```python
from build123d import *

# Parameters (mm, degrees)
EXTRUDE_1_DEPTH             = 30
FILLET_3_R                  = 3
SKETCH_9_R                  = 5
CUT_EXTRUDE_5_DEPTH         = 64.837130412
CUT_EXTRUDE_6_DEPTH         = 27
PATTERN_CIRCULAR_1_COUNT    = 3
SKETCH_11_W                 = 20
SKETCH_11_H                 = 0.244863729
CUT_EXTRUDE_7_DEPTH         = 64.837130412
CUT_EXTRUDE_8_REACH         = 74.953
SKETCH_12_R                 = 1.5
HOLE_WIZARD_M3_1_AT_2_COUNT = 2
HOLE_WIZARD_M3_1_AT_2_PITCH = 24
PATTERN_CIRCULAR_2_COUNT    = 3
SKETCH_15_R                 = 2
CUT_EXTRUDE_9_DEPTH         = 64.630599801


with BuildPart() as part:
    # Sketch 1 → Extrude 1 (new body)
    with BuildSketch(Plane(origin=(0, 0, 0), x_dir=(1, 0, 0), z_dir=(0, 1, 0))):
        Polygon((33, 25.3), (13, 25.3), (13, 22.051270189), (-27.806079661, 22.051270189), (-38.410442716, 15.928838325), (-28.410442716, -1.391669751), (-25.59696017, 0.232695155), (-5.193920339, -35.106406461), (5.410442716, -41.228838325), (15.410442716, -23.908330249), (12.59696017, -22.283965344), (33, 13.055136271), align=None)
    extrude(amount=EXTRUDE_1_DEPTH)

    # Fillet 3
    fillet_3_edges = [part.edges().sort_by_distance(p)[0] for p in [
        (13, 15, -22.051270189),
        (12.59696017, 15, 22.283965344),
        (-25.59696017, 15, -0.232695155),
    ]]
    fillet(fillet_3_edges, radius=FILLET_3_R)

    # Sketch 9 → Cut-Extrude 5 (cut, through all)
    with BuildSketch(Plane.XZ):
        with Locations(Location((0, 0, 0), (0, 0, 270))):
            Circle(SKETCH_9_R)
    extrude(amount=-CUT_EXTRUDE_5_DEPTH, mode=Mode.SUBTRACT)

    # Sketch 10 → Cut-Extrude 6 (cut)
    with BuildSketch(Plane.XZ):
        with BuildLine():
            Line((-27.806079661, -22.051270189), (-17.556079661, -4.297749412))
            ThreePointArc((-17.556079661, -4.297749412), (-15.734460585, -2.899971933), (-13.458003449, -3.1996732))
            Line((-13.458003449, -3.1996732), (11.5, -17.60918321))
            ThreePointArc((11.5, -17.60918321), (12.598076211, -18.707259422), (13, -20.207259422))
            Line((13, -20.207259422), (13, -25.051270189))
            Line((13, -25.051270189), (-27.806079661, -22.051270189))
        make_face()
    cut_extrude_6 = extrude(amount=-CUT_EXTRUDE_6_DEPTH, mode=Mode.SUBTRACT)

    # Pattern Circular 1: Cut-Extrude 6 ×3 about axis
    pattern_circular_1_axis = Axis((0, 0, 0), (0, 1, 0))
    for i in range(1, PATTERN_CIRCULAR_1_COUNT):
        add(cut_extrude_6.rotate(pattern_circular_1_axis, i * 360 / PATTERN_CIRCULAR_1_COUNT), mode=Mode.SUBTRACT)

    # Sketch 11 → Cut-Extrude 7 (cut, through all)
    with BuildSketch(Plane.XZ):
        with Locations((23, -25.177568136)):
            Rectangle(SKETCH_11_W, SKETCH_11_H)
    cut_extrude_7 = extrude(amount=-CUT_EXTRUDE_7_DEPTH, mode=Mode.SUBTRACT)

    # Sketch 12 → Cut-Extrude 8 (cut, up to next)
    with BuildSketch(Plane(origin=(0, 0, -13.055136271), x_dir=(-1, 0, 0), z_dir=(0, 0, -1)), mode=Mode.PRIVATE) as cut_extrude_8_sk1:
        with Locations(Location((-30.5, 10, 0), (0, 0, 180))):
            Circle(SKETCH_12_R)
    cut_extrude_8_tool1 = extrude(cut_extrude_8_sk1.sketch, amount=CUT_EXTRUDE_8_REACH, mode=Mode.PRIVATE) & part.part
    # Sketch 12 → Cut-Extrude 8 (cut, up to next)
    with BuildSketch(Plane(origin=(0, 0, -13.055136271), x_dir=(-1, 0, 0), z_dir=(0, 0, -1)), mode=Mode.PRIVATE) as cut_extrude_8_sk2:
        with Locations(Location((-30.5, 20, 0), (0, 0, 180))):
            Circle(SKETCH_12_R)
    cut_extrude_8_tool2 = extrude(cut_extrude_8_sk2.sketch, amount=CUT_EXTRUDE_8_REACH, mode=Mode.PRIVATE) & part.part
    # Sketch 12 → Cut-Extrude 8 (cut, up to next)
    with BuildSketch(Plane(origin=(0, 0, -13.055136271), x_dir=(-1, 0, 0), z_dir=(0, 0, -1)), mode=Mode.PRIVATE) as cut_extrude_8_sk3:
        with Locations(Location((-15.5, 20, 0), (0, 0, 180))):
            Circle(SKETCH_12_R)
    cut_extrude_8_tool3 = extrude(cut_extrude_8_sk3.sketch, amount=CUT_EXTRUDE_8_REACH, mode=Mode.PRIVATE) & part.part
    # Sketch 12 → Cut-Extrude 8 (cut, up to next)
    with BuildSketch(Plane(origin=(0, 0, -13.055136271), x_dir=(-1, 0, 0), z_dir=(0, 0, -1)), mode=Mode.PRIVATE) as cut_extrude_8_sk4:
        with Locations(Location((-15.5, 10, 0), (0, 0, 180))):
            Circle(SKETCH_12_R)
    cut_extrude_8_tool4 = extrude(cut_extrude_8_sk4.sketch, amount=CUT_EXTRUDE_8_REACH, mode=Mode.PRIVATE) & part.part
    cut_extrude_8_1 = cut_extrude_8_tool1.solids().sort_by_distance((30.5, 10, -13.055136))[0]
    add(cut_extrude_8_1, mode=Mode.SUBTRACT)
    cut_extrude_8_2 = cut_extrude_8_tool2.solids().sort_by_distance((30.5, 20, -13.055136))[0]
    add(cut_extrude_8_2, mode=Mode.SUBTRACT)
    cut_extrude_8_3 = cut_extrude_8_tool3.solids().sort_by_distance((15.5, 20, -13.055136))[0]
    add(cut_extrude_8_3, mode=Mode.SUBTRACT)
    cut_extrude_8_4 = cut_extrude_8_tool4.solids().sort_by_distance((15.5, 10, -13.055136))[0]
    add(cut_extrude_8_4, mode=Mode.SUBTRACT)
    cut_extrude_8 = cut_extrude_8_1 + cut_extrude_8_2 + cut_extrude_8_3 + cut_extrude_8_4  # Cut-Extrude 8 as one shape, for the pattern or mirror that repeats it

    # Sketch 14 → Hole Wizard M3 _1 (revolve, cut)
    with BuildSketch(Plane(origin=(33, 3, -19.055136271), x_dir=(0, 0, -1), z_dir=(0, 1, 0))):
        Polygon((0, 0), (0, 8.251075774), (1.25, 7.5), (1.25, 0.275), (1.525, 0), align=None)
    hole_wizard_m3_1 = revolve(axis=Axis((39.35, 3, -19.055136271), (-1, 0, 0)), mode=Mode.SUBTRACT)

    # Hole Wizard M3 _1 at 2: Hole Wizard M3 _1 ×2
    with Locations(*[(0, i * HOLE_WIZARD_M3_1_AT_2_PITCH, 0) for i in range(1, HOLE_WIZARD_M3_1_AT_2_COUNT)]):
        add(hole_wizard_m3_1, mode=Mode.SUBTRACT)

    # Pattern Circular 2: Cut-Extrude 7, Cut-Extrude 8, Hole Wizard M3 _1 ×3 about axis
    pattern_circular_2_axis = Axis((0, 0, 0), (0, 1, 0))
    add([cut_extrude_7.rotate(pattern_circular_2_axis, i * 360 / PATTERN_CIRCULAR_2_COUNT) for i in range(1, PATTERN_CIRCULAR_2_COUNT)], mode=Mode.SUBTRACT)
    add([cut_extrude_8.rotate(pattern_circular_2_axis, i * 360 / PATTERN_CIRCULAR_2_COUNT) for i in range(1, PATTERN_CIRCULAR_2_COUNT)], mode=Mode.SUBTRACT)
    add([hole_wizard_m3_1.rotate(pattern_circular_2_axis, i * 360 / PATTERN_CIRCULAR_2_COUNT) for i in range(1, PATTERN_CIRCULAR_2_COUNT)], mode=Mode.SUBTRACT)

    # Pattern Circular 2 copy 1 sketch → Pattern Circular 2 copy 1 (revolve, cut)
    with BuildSketch(Plane(origin=(-33.002232084, 27, -19.051270189), x_dir=(-0.8660254037844396, 0, 0.4999999999999983), z_dir=(0, 1, 0))):
        Polygon((0, 0), (0, 8.251075774), (1.25, 7.5), (1.25, 0.275), (1.525, 0), align=None)
    revolve(axis=Axis((-36.177232084, 27, -24.550531503), (0.4999999999999983, 0, 0.8660254037844396)), mode=Mode.SUBTRACT)

    # Pattern Circular 2 copy 2 sketch → Pattern Circular 2 copy 2 (revolve, cut)
    with BuildSketch(Plane(origin=(0.002232084, 27, 38.106406461), x_dir=(0.8660254037844375, 0, 0.5000000000000019), z_dir=(0, 1, 0))):
        Polygon((0, 0), (0, 8.251075774), (1.25, 7.5), (1.25, 0.275), (1.525, 0), align=None)
    revolve(axis=Axis((-3.172767916, 27, 43.605667775), (0.5000000000000019, 0, -0.8660254037844375)), mode=Mode.SUBTRACT)

    # Sketch 15 → Cut-Extrude 9 (cut, through all)
    with BuildSketch(Plane(origin=(0, 30, 0), x_dir=(1, 0, 0), z_dir=(0, 1, 0))):
        with Locations(Location((-8.90303983, 18.051270189, 0), (0, 0, 270))):
            Circle(SKETCH_15_R)
        with Locations(Location((20.08437847, -1.315376431, 0), (0, 0, 270))):
            Circle(SKETCH_15_R)
        with Locations(Location((-11.181338639, -16.735893759, 0), (0, 0, 270))):
            Circle(SKETCH_15_R)
    extrude(amount=-CUT_EXTRUDE_9_DEPTH, mode=Mode.SUBTRACT)


solid = part.part
```
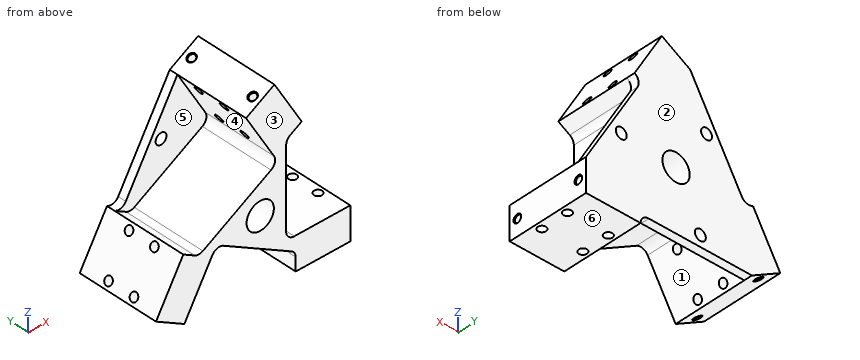
Part model, mm, in its own coordinate system. Face numbers are marked on the shaded views. A direction names the side the tool comes from. Round coordinates to 2 decimals unless told otherwise and drop trailing zeros. Order: outer loops, then holes, each group sorted by start corner. A loop starts at its lowest first (then second) coordinate and runs counter-clockwise, first axis right, second up. Notation, with made-up numbers: M -40,84 L -28,84 A15 ccw -28,97 Z; hole C 7.5,-29.5 d8. An arc over 180 degrees is marked long. Answer in a Markdown table with one row per item. Add a question column.
Q1. Mould opens along Z. For the marked faces 3, 4, 5 and 6 say: +Z half, -Z half, draft (parallel to the pull), parting line (faces both ways), or undercut.
Q2. Cut at C-C on x = 30.5. Give the cut face in (y, z) (3 decimals), and give its area (3 significant figures).
Q3. Cut at B-B on x = -8. Give the cut face in (y, z), and give its area (3 significant figures).
Q4. Wall check: L1, parallel to Y at x = 15.5, z = -21.5; L2, parallel to Z at x = 19, y = 21; L3, parallel to Y at x = -4.5, z = 15. Give the ranges that are in metal, low to high. Write a range as from..to.
Q5. 3-axis set-ups, long thin cutter, end or side, ignore diameter. For the marked faces 1 and 2: which of +Z, -Z, +X, -X, +Y, -Y reach the whole face in a straight line?
Q6. Pin check, flat tips, straight feed: pin 1 (5.5 mm diameter, centred on y = 15.5, z = -23, fed in from -X); pin 2 (4 mm diameter, centred on x = -3.5, y = 21, fed in from -Z); pin 3 (2 mm diameter, centred on x = -14, y = 9.5, fed in from -Z); pin 4 (3 mm diameter, centred on x = -8.9, z = -18.05, fed in from +Y). Stop position of each tip, or through.
Q7. Cut at A-A on y = 15. Give the cut face in (x, z).
Q8. Cut at D-D on y = 10. Give the number of separate pieces and of enclosed holes in the cut face, and give its area (3 significant figures).
Established:
| question | item | result |
|---|---|---|
| 1 | face 3 | draft |
| 1 | face 4 | undercut |
| 1 | face 5 | undercut |
| 1 | face 6 | -Z half |
| 2 | outline | M 0,-25.055 L 8.5,-25.055 L 8.5,-13.055 L 0,-13.055 Z; M 11.5,-25.055 L 18.5,-25.055 L 18.5,-13.055 L 11.5,-13.055 Z; M 21.5,-25.055 L 30,-25.055 L 30,-8.725 L 27,-8.725 L 27,-13.055 L 21.5,-13.055 Z; hole C 3,-19.055 d2.5; hole C 27,-19.055 d2.5 |
| 2 | area | 291 mm2 |
| 3 | outline | M 0,-6.35 L 27,-6.35 L 27,-16.27 L 30,-16.27 L 30,30.25 L 27,30.25 L 27,6.35 L 0,6.35 Z; M 27,-22.05 L 30,-22.05 L 30,-19.84 L 27,-19.84 Z |
| 3 | area | 489 mm2 |
| 4 | L1 | y = 0..8.5, 11.5..18.5, 21.5..30 |
| 4 | L2 | z = -25.06..-13.06 |
| 4 | L3 | y = 27..30 |
| 5 | face 1 | -Z, -Y |
| 5 | face 2 | +Z, -Z, +X, -X, +Y |
| 6 | pin 1 | stops at x = -30.93 |
| 6 | pin 2 | stops at z = -10.1 |
| 6 | pin 3 | stops at z = -3.46 |
| 6 | pin 4 | passes through |
| 7 | outline | M -38.2,-16.05 L -27.81,-22.05 L -17.56,-4.3 A3 cw -13.46,-3.2 L 11.5,-17.61 A3 cw 13,-20.21 L 13,-25.06 L 33,-25.06 L 33,-13.06 L 12.5,-13.06 A3 cw 9.5,-10.06 L 9.5,18.76 A3 cw 11,21.36 L 15.2,23.79 L 5.2,41.11 L -5.19,35.11 L 5.06,17.35 A3 cw 3.96,13.25 L -21,-1.15 A3 cw -24,-1.15 L -28.2,1.27 Z; hole C 0,0 d10 |
| 8 | separate pieces | 7 |
| 8 | enclosed holes | 1 |
| 8 | area | 948 mm2 |
